Autodesk Inventor part; units mm, degrees
ref_plane "Work Plane1" through (29, 0, 0) normal (0, -1, 0) x (1, 0, 0)
ref_plane "YZ Plane" through (0, 0, 0) normal (1, 0, 0) x (0, 1, 0)
ref_plane "XZ Plane" through (0, 0, 0) normal (0, 1, 0) x (-1, 0, 0)
sketch "Sketch1" plane through (0, 0, 0) normal (0, 0, 1) x (1, 0, 0)
  line L0 (-1.7145, 0) -> (127, 0)
  line L1 (127, 0) -> (127, 3.175)
  line L2 (127, 3.175) -> (101.6, 3.175)
  line L3 (101.6, 3.175) -> (99.0599, 3.175)
  line L4 (99.0599, 3.175) -> (0, 3.175)
  line L5 (0, 3.175) -> (0, 4.7625)
  line L6 (0, 4.7625) -> (-6.35, 4.7625)
  line L7 (-6.35, 4.7625) -> (-6.35, 2.7496)
  line L8 (-6.35, 2.7496) -> (-3.302, 2.7496)
  line L9 (-3.302, 2.7496) -> (-1.7145, 0)
  line L10 (-33.02, 0) -> (153.67, 0)
  line L11 (0, -0.9525) -> (0, 5.715)
  line L12 (101.6, 3.175) -> (0, 3.175) construction
  dimension "d1" = 25.4
  dimension "d2" = 2.5401
  dimension "d3" = 6.35
  dimension "d4" = 3.048
  dimension "d5" = 60
  dimension "d6" = 6.35
  dimension "d7" = 6.35
  dimension "d8" = 5.4993
  dimension "d9" = 9.525
  dimension "d26" = 127
revolve "Body" add sketch "Sketch1" angle 360 about axis through (-1.7145, 0, 0) along (1, 0, 0)
sketch "Sketch2" plane through (-6.35, 0, 0) normal (-1, 0, 0) x (0, 0, 1)
  circle A0 centre (0, 0) radius 2.7496
  line L0 (0, -6.6675) -> (0, 6.6675)
  line L1 (-6.6675, 0) -> (6.6675, 0)
  line L2 (2.7496, 0) -> (1.3748, -2.3812)
  line L3 (1.3748, -2.3812) -> (-1.3748, -2.3813)
  line L4 (-1.3748, -2.3813) -> (-2.7496, 0)
  line L5 (-2.7496, 0) -> (-1.3748, 2.3812)
  line L6 (-1.3748, 2.3812) -> (1.3748, 2.3813)
  line L7 (1.3748, 2.3813) -> (2.7496, 0)
extrude "Slot" add sketch "Sketch2" against normal up to next contours L7 A0 | A0 L2 | L6 L0 A0 | A0 L0 L3 | L0 L6 A0 | A0 L3 L0 | L4 A0 | A0 L5
fillet "Fillet1" radius 0.3556 1 edges at (-6.35, -4.7625, 0)
thread "Thread"
chamfer "Chamfer1" distance 0.7791 distance2 0.779 1 edges at (127, -3.175, 0) measured on face at (127, 0.9371, 0.4918)
ref_plane "Work Plane1" through (29, 0, 0) normal (0, -1, 0) x (1, 0, 0)
fillet "Fillet2" radius 0.1 1 edges at (0, -3.175, 0)
equation "\"d30\" = R"
equation "\"d17\" = RR"
equation "\"d13\" = GEL"
equation "\"d15\" = -0.5 * SPD + 0.5 * GD"
equation "\"d16\" = GUL"
equation "\"d1\" = GEL"
equation "\"d3\" = KOH"
equation "\"d4\" = INTI"
equation "\"d6\" = GD"
equation "\"d7\" = BDM"
equation "\"d8\" = 1.1547 * SW"
equation "\"d9\" = KOD"
equation "\"d26\" = NLG"
equation "\"GD\" = NND"
equation "\"NLG\" = 127"
equation "\"GEL\" = 25.4"
equation "\"KOD\" = 9.525"
equation "\"KOH\" = NND"
equation "\"INTI\" = 3.048"
equation "\"GAL\" = 2.54"
equation "\"GUL\" = 0.77902"
equation "\"BDM\" = NND"
equation "\"SW\" = 4.7625"
equation "\"RR\" = 0.3556"
equation "\"SPD\" = GD1"
equation "\"R\" = 0.1"
equation "\"PHH\" = 0.1 * NND"
equation "\"THREADDIA\" = 6.35"
equation "\"FAWI\" = 45deg"
equation "\"NND\" = 6.35"
equation "\"E0\" = 1.155 * SW"
equation "\"FAWI1\" = 30deg"
equation "\"TOA\" = 30deg"
equation "\"GD1\" = 4.79189"
properties part number "Unbrako - 1/4 x 5" material "Steel, Mild"
Design review of the part built by this model. Coordinates are the model's own, in mm. A direction names the side the tool comes from. Round coordinates to 2 decimals unless told otherwise and drop trailing zeros. Write each loop counter-clockwise with the first axis right and the second up, starting at its lowest first coordinate (ties: lowest second). Pieces come first, ordered by that corner, then holes. Notation, with made-up numbers: (45.5, -19.75) -> (62.5, -19.75) arc R31 ccw to (62.5, 8.25) -> close; hole circle Ø7 at (25, -23). An arc over 180 degrees is marked (long way). One line per question, with ' | ' between items.
(1) Wall thickness on line 1 (X direction, y = 2, z = -3.5); line 2 (Z direction, x = 78.5, y = -0.25); line 3 (Y direction, x = 46, z = 1.25): over which ranges is each line inside the solid? List them lowest first. Write a range as [from, to].
Result sheet:
line 1: [-6.35, 0] | line 2: [-3.17, 3.17] | line 3: [-2.92, 2.92]
(2) Take a section at A-A, the plane x = 9. State the section outline as (y, z) points (3 decimals).
Result sheet:
outline: circle Ø6.35 at (0, 0)
(3) Insertion check: P1, Ø2, axis at x = 22.5, y = -1, coming from the +Z side (3 decimals); P2, Ø5, axis at x = 49, y = 3, coming from the -Z side; P3, Ø1, axis at x = 29, y = 0, coming from the -Z side (3 decimals). Each pin has a flat end and moves straight along its axis. Give the tip position at first contact, or say it passes through.
Result sheet:
P1: z = 3.175 | P2: z = -3.14 | P3: z = -3.175
(4) Machinability: for faces 1 (the flat face through (-4.742, -1.174, 2.072)), 2 (the cylindrical face through (62.28, -0.69, 3.1)), 3 (the flat face through (-6.35, -2, 2)), which of the approach directions +Z, -Z, +X, -X, +Y, -Y give a long, thin tool a straight path to every point of the face, cutting with its end or side? Answer none if there is none.
Result sheet:
face 1: -X | face 2: +X | face 3: +Z, -Z, -X, +Y, -Y
